Geometry: final body of the model. Coordinates: model frame, mm. A direction names the side the tool comes from. Give positions to 0.01 mm unless a question says otherwise; leave off trailing zeros. Order: outer loops, then holes, each group sorted by start corner. A loop starts at its lowest first (then second) coordinate and runs counter-clockwise, first axis right, second up. Notation, with made-up numbers: (-4, 57) -> (27, 57) arc R11 ccw to (27, 77) -> close; hole circle Ø5 at (-31, 23). An arc over 180 degrees is marked (long way). Write item = value, one per line.
```python
from build123d import *

# Parameters (mm, degrees)
SKETCH_1_W            = 109
SKETCH_1_H            = 57
EXTRUDE_1_DEPTH       = 2
CUT_EXTRUDE_1_DEPTH   = 3
MIRROR_2_COPY_1_DEPTH = 3
SKETCH_3_R            = 4
SKETCH_3_R_2          = 2.5
CUT_EXTRUDE_2_DEPTH   = 3
SKETCH_4_R            = 1.65
CUT_EXTRUDE_3_DEPTH   = 2
SKETCH_5_W            = 18
SKETCH_5_H            = 15
CUT_EXTRUDE_4_DEPTH   = 3
FILLET_1_R            = 1


with BuildPart() as part:
    # Эскиз1 → Бобышка-Вытянуть1 (new body)
    with BuildSketch(Plane(origin=(0, 0, 0), x_dir=(1, 0, 0), z_dir=(0, 1, 0))):
        Rectangle(SKETCH_1_W, SKETCH_1_H)
    extrude(amount=EXTRUDE_1_DEPTH)

    # Эскиз2 → Вырез-Вытянуть1 (cut, through all)
    with BuildSketch(Plane(origin=(0, 2, 0), x_dir=(1, 0, 0), z_dir=(0, 1, 0))):
        Polygon((49.4, 19.5), (54.5, 19.5), (54.5, 28.5), (47, 28.5), (47, 23.9), (49.4, 23.9), align=None)
    cut_extrude_1 = extrude(amount=-CUT_EXTRUDE_1_DEPTH, mode=Mode.SUBTRACT)

    # Зеркальное отражение1: Вырез-Вытянуть1 across plane
    add(cut_extrude_1.mirror(Plane(origin=(0, 0, 0), x_dir=(0, 0, 1), z_dir=(1, 0, 0))), mode=Mode.SUBTRACT)

    # Зеркальное отражение2: Вырез-Вытянуть1 across plane
    add(cut_extrude_1.mirror(Plane.XY), mode=Mode.SUBTRACT)

    # Зеркальное отражение2 copy 1 sketch → Зеркальное отражение2 copy 1 (cut, through all)
    with BuildSketch(Plane(origin=(0, 2, 0), x_dir=(-1, 0, 0), z_dir=(0, 1, 0))):
        Polygon((49.4, 19.5), (54.5, 19.5), (54.5, 28.5), (47, 28.5), (47, 23.9), (49.4, 23.9), align=None)
    extrude(amount=-MIRROR_2_COPY_1_DEPTH, mode=Mode.SUBTRACT)

    # Эскиз3 → Вырез-Вытянуть2 (cut, through all)
    with BuildSketch(Plane(origin=(0, 2, 0), x_dir=(1, 0, 0), z_dir=(0, 1, 0))):
        with Locations((-33.9, -12.75)):
            Circle(SKETCH_3_R)
        with Locations((32.1, -12.75)):
            Circle(SKETCH_3_R_2)
    extrude(amount=-CUT_EXTRUDE_2_DEPTH, mode=Mode.SUBTRACT)

    # Эскиз4 → Вырез-Вытянуть3 (cut)
    with BuildSketch(Plane(origin=(0, 2, 0), x_dir=(1, 0, 0), z_dir=(0, 1, 0))):
        with Locations((17.16, -10.2)):
            Circle(SKETCH_4_R)
        with Locations((-16.16, -10.2)):
            Circle(SKETCH_4_R)
        with BuildLine():
            Line((-11.5, -5.2), (12.5, -5.2))
            ThreePointArc((12.5, -5.2), (13.914213562, -5.785786438), (14.5, -7.2))
            Line((14.5, -7.2), (14.5, -13.2))
            ThreePointArc((14.5, -13.2), (13.914213562, -14.614213562), (12.5, -15.2))
            Line((12.5, -15.2), (-11.5, -15.2))
            ThreePointArc((-11.5, -15.2), (-12.914213562, -14.614213562), (-13.5, -13.2))
            Line((-13.5, -13.2), (-13.5, -7.2))
            ThreePointArc((-13.5, -7.2), (-12.914213562, -5.785786438), (-11.5, -5.2))
        make_face()
    extrude(amount=-CUT_EXTRUDE_3_DEPTH, mode=Mode.SUBTRACT)

    # Эскиз5 → Вырез-Вытянуть4 (cut, through all)
    with BuildSketch(Plane(origin=(0, 2, 0), x_dir=(1, 0, 0), z_dir=(0, 1, 0))):
        with Locations((4.5, 13.25)):
            Rectangle(SKETCH_5_W, SKETCH_5_H)
    extrude(amount=-CUT_EXTRUDE_4_DEPTH, mode=Mode.SUBTRACT)

    # Эскиз6 → Зенковка для винта с полупотайной головкой M31 (revolve, cut)
    with BuildSketch(Plane(origin=(37.5, 2, -25.25), x_dir=(0, 0, 1), z_dir=(1, 0, 0))):
        Polygon((0, 0), (0, 2.001), (1.7, 2.001), (1.7, 1.45), (3.15, 0), align=None)
    hole_wizard_m31 = revolve(axis=Axis((37.5, 8.35, -25.25), (0, -1, 0)), mode=Mode.SUBTRACT)

    # Зеркальное отражение3: Зенковка для винта с полупотайной головкой M31 across plane
    add(hole_wizard_m31.mirror(Plane.XY), mode=Mode.SUBTRACT)

    # Зеркальное отражение4: Зенковка для винта с полупотайной головкой M31 across plane
    add(hole_wizard_m31.mirror(Plane(origin=(0, 0, 0), x_dir=(0, 0, 1), z_dir=(1, 0, 0))), mode=Mode.SUBTRACT)

    # Зеркальное отражение4 copy 1 sketch → Зеркальное отражение4 copy 1 (revolve, cut)
    with BuildSketch(Plane(origin=(-37.5, 2, 25.25), x_dir=(0, 0, -1), z_dir=(-1, 0, 0))):
        Polygon((0, 0), (0, 2.001), (1.7, 2.001), (1.7, 1.45), (3.15, 0), align=None)
    revolve(axis=Axis((-37.5, 8.35, 25.25), (0, -1, 0)), mode=Mode.SUBTRACT)

    # Скругление1
    fillet_1_edges = [part.edges().sort_by_distance(p)[0] for p in [
        (13.5, 1, -20.75),
        (13.5, 1, -5.75),
        (-4.5, 1, -5.75),
        (-4.5, 1, -20.75),
    ]]
    fillet(fillet_1_edges, radius=FILLET_1_R)


solid = part.part
```
1) Section query A-A (x = 37.5). Output: boundary loops of the cut face in (y, z).
Check sheet entries:
outline = (0, -28.5) -> (2, -28.5) -> (2, -28.4) -> (0.55, -26.95) -> (0, -26.95) -> close; (0, -23.55) -> (0.55, -23.55) -> (2, -22.1) -> (2, 22.1) -> (0.55, 23.55) -> (0, 23.55) -> close; (0, 26.95) -> (0.55, 26.95) -> (2, 28.4) -> (2, 28.5) -> (0, 28.5) -> close
2) Line query: line 1 (X direction, y = 0.5, z = 12.75); line 2 (X direction, y = 0.25, z = -25.25); line 3 (Z direction, x = 37.5, y = 0.4). Output: solid intervals per line, ascending. Write a range as from..to.
Check sheet entries:
line_1 = -54.5..-37.9, -29.9..-13.5, 14.5..29.6, 34.6..54.5
line_2 = -47..-39.2, -35.8..35.8, 39.2..47
line_3 = -28.5..-26.95, -23.55..23.55, 26.95..28.5
3) Section query D-D (x = 1). Output: boundary loops of the cut face in (y, z).
Check sheet entries:
outline = (0, -28.5) -> (2, -28.5) -> (2, -20.75) -> (0, -20.75) -> close; (0, -5.75) -> (2, -5.75) -> (2, 5.2) -> (0, 5.2) -> close; (0, 15.2) -> (2, 15.2) -> (2, 28.5) -> (0, 28.5) -> close
4) Mould query, pull axis Z, two halves, no side actions, for faces 5 (the face through (-12.9, 1.01, 14.63)), 6 (the face through (-52, 1, -19.5)), 7 (the face through (49.4, 1, -22)). Classes: +Z half, -Z half, draft (parallel to the pull), parting line (faces both ways), or undercut.
Check sheet entries:
face_5 = undercut
face_6 = -Z half
face_7 = draft
5) First-contact query: P1, Ø1, axis at y = 1, z = -22, coming from the -X side; P2, Ø1, axis at y = 1, z = -25, coming from the -X side; P3, Ø0.6, axis at y = 0.5, z = -26, coming from the +X side. Flat tips, straight axial feed; report the tip coordinate or a pass-through.
Check sheet entries:
P1 = -49.4
P2 = -47
P3 = 47
6) Section query B-B (z = -25.25). Output: boundary loops of the cut face in (x, y).
Check sheet entries:
outline = (-47, 0) -> (-39.2, 0) -> (-39.2, 0.55) -> (-40.65, 2) -> (-47, 2) -> close; (-35.8, 0) -> (35.8, 0) -> (35.8, 0.55) -> (34.35, 2) -> (-34.35, 2) -> (-35.8, 0.55) -> close; (39.2, 0) -> (47, 0) -> (47, 2) -> (40.65, 2) -> (39.2, 0.55) -> close
7) Section query C-C (x = 17.16). Output: boundary loops of the cut face in (y, z), plus the area to 3 significant figures.
Check sheet entries:
outline = (0, -28.5) -> (2, -28.5) -> (2, 8.55) -> (0, 8.55) -> close; (0, 11.85) -> (2, 11.85) -> (2, 28.5) -> (0, 28.5) -> close
area = 107 mm²
8) Reachability of faces 1 (the face through (-48, 1, -23.9)), 2 (the face through (48, 1, 23.9)), 3 (the face through (-1, 2, 0)), 4 (the face through (-12.93, 1.01, 5.8)) from +Z, -Z, +X, -X, +Y, -Y: full face, straight path, thin tool, end or side. Return the list, or none.
Check sheet entries:
face_1 = -Z, -X, +Y, -Y
face_2 = +Z, +X, +Y, -Y
face_3 = +Z, -Z, +X, -X, +Y
face_4 = +Y, -Y
